from build123d import *

# Parameters (mm, degrees)
AUFSATZ_LINEAR_AUSTRAGEN1_DEPTH = 2
SKIZZE3_R                       = 2.35
SCHNITT_LINEAR_AUSTRAGEN1_DEPTH = 109.995412748


with BuildPart() as part:
    # Skizze1 → Aufsatz-Linear austragen1 (new body)
    with BuildSketch(Plane.XY):
        with BuildLine():
            Line((-35, 49), (35, 49))
            ThreePointArc((35, 49), (52.67766953, 56.32233047), (60, 74))
            Line((60, 74), (80, 74))
            Line((80, 74), (80, -74))
            Line((80, -74), (-80, -74))
            Line((-80, -74), (-80, 74))
            Line((-80, 74), (-60, 74))
            ThreePointArc((-60, 74), (-52.67766953, 56.32233047), (-35, 49))
        make_face()
    extrude(amount=AUFSATZ_LINEAR_AUSTRAGEN1_DEPTH)

    # Skizze3 → Schnitt-Linear austragen1 (cut, through all)
    with BuildSketch(Plane.XY.offset(2)):
        with Locations((71, 65)):
            Circle(SKIZZE3_R)
        with Locations((-71, -65)):
            Circle(SKIZZE3_R)
        with Locations((71, -65)):
            Circle(SKIZZE3_R)
        with Locations((-71, 65)):
            Circle(SKIZZE3_R)
    extrude(amount=-SCHNITT_LINEAR_AUSTRAGEN1_DEPTH, mode=Mode.SUBTRACT)


solid = part.part
CAD build for the part. Positions are in the model's coordinates, mm. A direction names the side the tool comes from. Coordinates: 2 decimals unless noted, no trailing zeros. Write each loop counter-clockwise with the first axis right and the second up, starting at its lowest first coordinate (ties: lowest second). Pieces come first, ordered by that corner, then holes. Notation, with made-up numbers: (4, 45.5) - (23, 45.5) arc R21 cw to (23, 78.5) - close; hole circle Ø3 at (33, 78.25). An arc over 180 degrees is marked (long way). Use a Markdown table: item, result. Add a question column.
Item 1: Band-saw the part on D-D, the plane x = -13. Give the cut face in (y, z).
Item 2: Mould opens along X. For faces 3 (the face through (-71.31, -62.67, 1.01)), 4 (the face through (1, -15, 2)) say: pulls with the +X half, pulls with the -X half, needs draft (parallel to the pull), parting line crosses it, or undercut.
Item 3: Flat gauge pin, fed straight in: pin 1 (3 mm diameter, centred on x = 71, y = -65, fed in from +Z). Where does the tip first touch, or does it go through?
Item 4: 3-axis set-ups, long thin cutter, end or side, ignore diameter. For faces 1 (the face through (52.482, 56.129, 0.986)), 2 (the face through (1, -15, 0)): which of +Z, -Z, +X, -X, +Y, -Y reach the whole face in a straight line?
Item 5: Band-saw the part on C-C, the plane y = 65. Give the cut face in (x, z), and give its area (3 significant figures).
Item 6: Band-saw the part on B-B, the plane z = 1.55. Give the cut face in (x, y), and give its area (3 significant figures).
Item 7: Drill centre lines: L1, parallel to Y at x = 71, z = 1.1; L2, parallel to X at y = -66, z = 0.95; L3, parallel to X at y = 58.5, z = 1.85. Where is each one in solid material? Low to high. Write a range as from..to.
Item 8: Band-saw the part on A-A, the plane x = -71. Give the cut face in (y, z).
Numbers:
| question | item | result |
|---|---|---|
| 1 | outline | (-74, 0) - (49, 0) - (49, 2) - (-74, 2) - close |
| 2 | face 3 | undercut |
| 2 | face 4 | needs draft |
| 3 | pin 1 | through |
| 4 | face 1 | +Z, -Z, +Y |
| 4 | face 2 | -Z, +X, -X, +Y, -Y |
| 5 | outline | (-80, 0) - (-73.35, 0) - (-73.35, 2) - (-80, 2) - close; (-68.65, 0) - (-58.32, 0) - (-58.32, 2) - (-68.65, 2) - close; (58.32, 0) - (68.65, 0) - (68.65, 2) - (58.32, 2) - close; (73.35, 0) - (80, 0) - (80, 2) - (73.35, 2) - close |
| 5 | area | 67.9 mm2 |
| 6 | outline | (-80, -74) - (80, -74) - (80, 74) - (60, 74) arc R25 cw to (35, 49) - (-35, 49) arc R25 cw to (-60, 74) - (-80, 74) - close; hole circle Ø4.7 at (-71, -65); hole circle Ø4.7 at (-71, 65); hole circle Ø4.7 at (71, -65); hole circle Ø4.7 at (71, 65) |
| 6 | area | 20,900 mm2 |
| 7 | L1 | -74..-67.35, -62.65..62.65, 67.35..74 |
| 7 | L2 | -80..-73.13, -68.87..68.87, 73.13..80 |
| 7 | L3 | -80..-54.62, 54.62..80 |
| 8 | outline | (-74, 0) - (-67.35, 0) - (-67.35, 2) - (-74, 2) - close; (-62.65, 0) - (62.65, 0) - (62.65, 2) - (-62.65, 2) - close; (67.35, 0) - (74, 0) - (74, 2) - (67.35, 2) - close |
